Check sheet for the modelled part. Datum: model origin and axes. Units: mm. Coordinates: 2 decimals unless noted, no trailing zeros. Order: outer loops, then holes, each group sorted by start corner. A loop starts at its lowest first (then second) coordinate and runs counter-clockwise, first axis right, second up. Notation, with made-up numbers: M -28,-29 L 18,-29 A20 cw 18,-1 Z; hole C 12,69 d9. An arc over 180 degrees is marked long. Answer in a Markdown table with one row per item. Add a question column.
from build123d import *

# Parameters (mm, degrees)
CROQUIS1_W              = 50
CROQUIS1_H              = 138.4
CROQUIS1_R              = 4.7625
SALIENTE_EXTRUIR1_DEPTH = 9
CROQUIS2_R              = 2.5
CORTAR_EXTRUIR1_DEPTH   = 75.12583895
SALIENTE_EXTRUIR2_DEPTH = 9


with BuildPart() as part:
    # Croquis1 → Saliente-Extruir1 (new body)
    with BuildSketch(Plane(origin=(0, 0, 0), x_dir=(1, 0, 0), z_dir=(0, 1, 0))):
        Rectangle(CROQUIS1_W, CROQUIS1_H)
        with Locations(Location((0, 0, 0), (0, 0, 270))):
            Circle(CROQUIS1_R, mode=Mode.SUBTRACT)
    extrude(amount=SALIENTE_EXTRUIR1_DEPTH)

    # Croquis2 → Cortar-Extruir1 (cut, through all)
    with BuildSketch(Plane(origin=(0, 9, 0), x_dir=(1, 0, 0), z_dir=(0, 1, 0))):
        with Locations(Location((-15, -59.2, 0), (0, 0, 270))):
            Circle(CROQUIS2_R)
        with Locations(Location((15, -59.2, 0), (0, 0, 90))):
            Circle(CROQUIS2_R)
        with Locations(Location((15, 59.2, 0), (0, 0, 270))):
            Circle(CROQUIS2_R)
        with Locations(Location((-15, 59.2, 0), (0, 0, 90))):
            Circle(CROQUIS2_R)
    extrude(amount=-CORTAR_EXTRUIR1_DEPTH, mode=Mode.SUBTRACT)

    # Croquis3 → Saliente-Extruir2 (add)
    with BuildSketch(Plane(origin=(0, 9, 0), x_dir=(1, 0, 0), z_dir=(0, 1, 0))):
        Polygon((-25, 69.2), (-25, -69.2), (-35, -59.2), (-35, 59.2), align=None)
        Polygon((25, 69.2), (25, -69.2), (30, -60.539745962), (30, 60.539745962), align=None)
    extrude(amount=-SALIENTE_EXTRUIR2_DEPTH)


solid = part.part
1. Release check for a two-part mould opening along Z. For faces 1 (the cylindrical face through (15.96, 4.56, 56.89)), 2 (the flat face through (27.535, 4.563, -64.809)), 3 (the cylindrical face through (14.04, 4.56, -56.89)), 4 (the flat face through (-35, 5, 1)) record: released by +Z, released by -Z, zero draft, split by the parting line, or undercut.
2. Scan lines: line 1 (X direction, y = 4.5, z = -59.2); line 2 (X direction, y = 3.5, z = -58.5); line 3 (Z direction, x = -17, y = 1.75). Record each from-to range of solid material in increasing order.
3. Section check B-B on x = 15. Enter the section's corners in (y, z).
4. Section check D-D on x = 0. Enter the section's corners in (y, z).
5. Section check A-A on z = 0. Enter the section's corners in (x, y).
6. Section check C-C on y = 6.25. Enter the section's corners in (x, z) (1 decimal).
Result sheet:
| question | item | result |
|---|---|---|
| 1 | face 1 | undercut |
| 1 | face 2 | released by -Z |
| 1 | face 3 | undercut |
| 1 | face 4 | zero draft |
| 2 | line 1 | -35 to -17.5, -12.5 to 12.5, 17.5 to 30 |
| 2 | line 2 | -35 to -17.4, -12.6 to 12.6, 17.4 to 30 |
| 2 | line 3 | -69.2 to -60.7, -57.7 to 57.7, 60.7 to 69.2 |
| 3 | outline | M 0,-69.2 L 9,-69.2 L 9,-61.7 L 0,-61.7 Z; M 0,-56.7 L 9,-56.7 L 9,56.7 L 0,56.7 Z; M 0,61.7 L 9,61.7 L 9,69.2 L 0,69.2 Z |
| 4 | outline | M 0,-69.2 L 9,-69.2 L 9,-4.76 L 0,-4.76 Z; M 0,4.76 L 9,4.76 L 9,69.2 L 0,69.2 Z |
| 5 | outline | M -35,0 L -4.76,0 L -4.76,9 L -35,9 Z; M 4.76,0 L 30,0 L 30,9 L 4.76,9 Z |
| 6 | outline | M -35,-59.2 L -25,-69.2 L 25,-69.2 L 30,-60.5 L 30,60.5 L 25,69.2 L -25,69.2 L -35,59.2 Z; hole C -15,-59.2 d5; hole C -15,59.2 d5; hole C 0,0 d9.5; hole C 15,-59.2 d5; hole C 15,59.2 d5 |
